from build123d import *

# Parameters (mm, degrees)
SKETCH1_W           = 63.75
SKETCH1_H           = 36.5
BOSS_EXTRUDE1_DEPTH = 1
SKETCH2_W           = 63.75
SKETCH2_H           = 1
BOSS_EXTRUDE2_DEPTH = 15
BOSS_EXTRUDE3_DEPTH = 1
CUT_EXTRUDE1_REACH  = 18


with BuildPart() as part:
    # Sketch1 → Boss-Extrude1 (new body)
    with BuildSketch(Plane(origin=(0, 0, 0), x_dir=(1, 0, 0), z_dir=(0, 1, 0))):
        Rectangle(SKETCH1_W, SKETCH1_H)
    extrude(amount=-BOSS_EXTRUDE1_DEPTH)

    # Sketch2 → Boss-Extrude2 (add)
    with BuildSketch(Plane(origin=(0, -1, 0), x_dir=(-1, 0, 0), z_dir=(0, -1, 0))):
        with Locations((0, -17.75)):
            Rectangle(SKETCH2_W, SKETCH2_H)
    extrude(amount=BOSS_EXTRUDE2_DEPTH)

    # Sketch3 → Boss-Extrude3 (add)
    with BuildSketch(Plane.XY.offset(18.25)):
        Polygon((-31.875, 0), (31.875, 0), (31.875, -1), (29.875, -1), (29.875, -16), (-29.875, -16), (-29.875, -1), (-31.875, -1), align=None)
    extrude(amount=BOSS_EXTRUDE3_DEPTH)

    # Sketch4 → Cut-Extrude1 (cut, up to next)
    with BuildSketch(Plane(origin=(0, 0, 0), x_dir=(1, 0, 0), z_dir=(0, 1, 0)), mode=Mode.PRIVATE) as cut_extrude1_sk1:
        with BuildLine():
            Line((-23.706953695, -13.257748955), (-24.425558305, -12.539144346))
            ThreePointArc((-24.425558305, -12.539144346), (-25.839771867, -12.539144346), (-25.839771867, -13.953357908))
            Line((-25.839771867, -13.953357908), (-25.121167258, -14.671962518))
            ThreePointArc((-25.121167258, -14.671962518), (-23.706953695, -14.671962518), (-23.706953695, -13.257748955))
        make_face()
    cut_extrude1_tool1 = extrude(cut_extrude1_sk1.sketch, amount=-CUT_EXTRUDE1_REACH, mode=Mode.PRIVATE) & part.part
    add(cut_extrude1_tool1.solids().sort_by_distance((-24.773363, 0, 13.605553))[0], mode=Mode.SUBTRACT)
    # Sketch4 → Cut-Extrude1 (cut, up to next)
    with BuildSketch(Plane(origin=(0, 0, 0), x_dir=(1, 0, 0), z_dir=(0, 1, 0)), mode=Mode.PRIVATE) as cut_extrude1_sk2:
        with BuildLine():
            Line((-18.612300872, -13.743096131), (-24.910905481, -7.444491522))
            ThreePointArc((-24.910905481, -7.444491522), (-26.325119043, -7.444491522), (-26.325119043, -8.858705084))
            Line((-26.325119043, -8.858705084), (-20.026514434, -15.157309694))
            ThreePointArc((-20.026514434, -15.157309694), (-18.612300872, -15.157309694), (-18.612300872, -13.743096131))
        make_face()
    cut_extrude1_tool2 = extrude(cut_extrude1_sk2.sketch, amount=-CUT_EXTRUDE1_REACH, mode=Mode.PRIVATE) & part.part
    add(cut_extrude1_tool2.solids().sort_by_distance((-22.46871, 0, 11.300901))[0], mode=Mode.SUBTRACT)
    # Sketch4 → Cut-Extrude1 (cut, up to next)
    with BuildSketch(Plane(origin=(0, 0, 0), x_dir=(1, 0, 0), z_dir=(0, 1, 0)), mode=Mode.PRIVATE) as cut_extrude1_sk3:
        with BuildLine():
            Line((-12.983889235, -13.694684495), (-24.862493845, -1.816079885))
            ThreePointArc((-24.862493845, -1.816079885), (-26.276707407, -1.816079885), (-26.276707407, -3.230293448))
            Line((-26.276707407, -3.230293448), (-14.398102798, -15.108898057))
            ThreePointArc((-14.398102798, -15.108898057), (-12.983889235, -15.108898057), (-12.983889235, -13.694684495))
        make_face()
    cut_extrude1_tool3 = extrude(cut_extrude1_sk3.sketch, amount=-CUT_EXTRUDE1_REACH, mode=Mode.PRIVATE) & part.part
    add(cut_extrude1_tool3.solids().sort_by_distance((-19.630298, 0, 8.462489))[0], mode=Mode.SUBTRACT)
    # Sketch4 → Cut-Extrude1 (cut, up to next)
    with BuildSketch(Plane(origin=(0, 0, 0), x_dir=(1, 0, 0), z_dir=(0, 1, 0)), mode=Mode.PRIVATE) as cut_extrude1_sk4:
        with BuildLine():
            Line((-7.19192546, -13.482720719), (-24.650530069, 3.97588389))
            ThreePointArc((-24.650530069, 3.97588389), (-26.064743631, 3.97588389), (-26.064743631, 2.561670328))
            Line((-26.064743631, 2.561670328), (-8.606139022, -14.896934282))
            ThreePointArc((-8.606139022, -14.896934282), (-7.19192546, -14.896934282), (-7.19192546, -13.482720719))
        make_face()
    cut_extrude1_tool4 = extrude(cut_extrude1_sk4.sketch, amount=-CUT_EXTRUDE1_REACH, mode=Mode.PRIVATE) & part.part
    add(cut_extrude1_tool4.solids().sort_by_distance((-16.628335, 0, 5.460525))[0], mode=Mode.SUBTRACT)
    # Sketch4 → Cut-Extrude1 (cut, up to next)
    with BuildSketch(Plane(origin=(0, 0, 0), x_dir=(1, 0, 0), z_dir=(0, 1, 0)), mode=Mode.PRIVATE) as cut_extrude1_sk5:
        with BuildLine():
            Line((-1.598647721, -13.469442981), (-24.63725233, 9.569161629))
            ThreePointArc((-24.63725233, 9.569161629), (-26.051465893, 9.569161629), (-26.051465893, 8.154948066))
            Line((-26.051465893, 8.154948066), (-3.012861283, -14.883656543))
            ThreePointArc((-3.012861283, -14.883656543), (-1.598647721, -14.883656543), (-1.598647721, -13.469442981))
        make_face()
    cut_extrude1_tool5 = extrude(cut_extrude1_sk5.sketch, amount=-CUT_EXTRUDE1_REACH, mode=Mode.PRIVATE) & part.part
    add(cut_extrude1_tool5.solids().sort_by_distance((-13.825057, 0, 2.657247))[0], mode=Mode.SUBTRACT)
    # Sketch4 → Cut-Extrude1 (cut, up to next)
    with BuildSketch(Plane(origin=(0, 0, 0), x_dir=(1, 0, 0), z_dir=(0, 1, 0)), mode=Mode.PRIVATE) as cut_extrude1_sk6:
        with BuildLine():
            Line((3.848599736, -13.602195524), (-24.770004873, 15.016409086))
            ThreePointArc((-24.770004873, 15.016409086), (-26.184218436, 15.016409086), (-26.184218436, 13.602195524))
            Line((-26.184218436, 13.602195524), (2.434386174, -15.016409086))
            ThreePointArc((2.434386174, -15.016409086), (3.848599736, -15.016409086), (3.848599736, -13.602195524))
        make_face()
    cut_extrude1_tool6 = extrude(cut_extrude1_sk6.sketch, amount=-CUT_EXTRUDE1_REACH, mode=Mode.PRIVATE) & part.part
    add(cut_extrude1_tool6.solids().sort_by_distance((-11.167809, 0, 0))[0], mode=Mode.SUBTRACT)
    # Sketch4 → Cut-Extrude1 (cut, up to next)
    with BuildSketch(Plane(origin=(0, 0, 0), x_dir=(1, 0, 0), z_dir=(0, 1, 0)), mode=Mode.PRIVATE) as cut_extrude1_sk7:
        with BuildLine():
            Line((9.432504411, -13.602195524), (-19.186100198, 15.016409086))
            ThreePointArc((-19.186100198, 15.016409086), (-20.600313761, 15.016409086), (-20.600313761, 13.602195524))
            Line((-20.600313761, 13.602195524), (8.018290849, -15.016409086))
            ThreePointArc((8.018290849, -15.016409086), (9.432504411, -15.016409086), (9.432504411, -13.602195524))
        make_face()
    cut_extrude1_tool7 = extrude(cut_extrude1_sk7.sketch, amount=-CUT_EXTRUDE1_REACH, mode=Mode.PRIVATE) & part.part
    add(cut_extrude1_tool7.solids().sort_by_distance((-5.583905, 0, 0))[0], mode=Mode.SUBTRACT)
    # Sketch4 → Cut-Extrude1 (cut, up to next)
    with BuildSketch(Plane(origin=(0, 0, 0), x_dir=(1, 0, 0), z_dir=(0, 1, 0)), mode=Mode.PRIVATE) as cut_extrude1_sk8:
        with BuildLine():
            Line((15.016409086, -13.602195524), (-13.602195524, 15.016409086))
            ThreePointArc((-13.602195524, 15.016409086), (-15.016409086, 15.016409086), (-15.016409086, 13.602195524))
            Line((-15.016409086, 13.602195524), (13.602195524, -15.016409086))
            ThreePointArc((13.602195524, -15.016409086), (15.016409086, -15.016409086), (15.016409086, -13.602195524))
        make_face()
    cut_extrude1_tool8 = extrude(cut_extrude1_sk8.sketch, amount=-CUT_EXTRUDE1_REACH, mode=Mode.PRIVATE) & part.part
    add(cut_extrude1_tool8.solids().sort_by_distance((0, 0, 0))[0], mode=Mode.SUBTRACT)
    # Sketch4 → Cut-Extrude1 (cut, up to next)
    with BuildSketch(Plane(origin=(0, 0, 0), x_dir=(1, 0, 0), z_dir=(0, 1, 0)), mode=Mode.PRIVATE) as cut_extrude1_sk9:
        with BuildLine():
            Line((20.596409086, -13.602195524), (-8.022195524, 15.016409086))
            ThreePointArc((-8.022195524, 15.016409086), (-9.436409086, 15.016409086), (-9.436409086, 13.602195524))
            Line((-9.436409086, 13.602195524), (19.182195524, -15.016409086))
            ThreePointArc((19.182195524, -15.016409086), (20.596409086, -15.016409086), (20.596409086, -13.602195524))
        make_face()
    cut_extrude1_tool9 = extrude(cut_extrude1_sk9.sketch, amount=-CUT_EXTRUDE1_REACH, mode=Mode.PRIVATE) & part.part
    add(cut_extrude1_tool9.solids().sort_by_distance((5.58, 0, 0))[0], mode=Mode.SUBTRACT)
    # Sketch4 → Cut-Extrude1 (cut, up to next)
    with BuildSketch(Plane(origin=(0, 0, 0), x_dir=(1, 0, 0), z_dir=(0, 1, 0)), mode=Mode.PRIVATE) as cut_extrude1_sk10:
        with BuildLine():
            Line((26.184121966, -13.602099067), (-2.442291993, 15.016505543))
            ThreePointArc((-2.442291993, 15.016505543), (-3.856505543, 15.016312616), (-3.856312616, 13.602099067))
            Line((-3.856312616, 13.602099067), (24.770101343, -15.016505543))
            ThreePointArc((24.770101343, -15.016505543), (26.184314892, -15.016312616), (26.184121966, -13.602099067))
        make_face()
    cut_extrude1_tool10 = extrude(cut_extrude1_sk10.sketch, amount=-CUT_EXTRUDE1_REACH, mode=Mode.PRIVATE) & part.part
    add(cut_extrude1_tool10.solids().sort_by_distance((11.163905, 0, 0))[0], mode=Mode.SUBTRACT)
    # Sketch4 → Cut-Extrude1 (cut, up to next)
    with BuildSketch(Plane(origin=(0, 0, 0), x_dir=(1, 0, 0), z_dir=(0, 1, 0)), mode=Mode.PRIVATE) as cut_extrude1_sk11:
        with BuildLine():
            Line((26.184218436, -8.030004873), (3.137804476, 15.016409086))
            ThreePointArc((3.137804476, 15.016409086), (1.723590914, 15.016409086), (1.723590914, 13.602195524))
            Line((1.723590914, 13.602195524), (24.770004873, -9.444218436))
            ThreePointArc((24.770004873, -9.444218436), (26.184218436, -9.444218436), (26.184218436, -8.030004873))
        make_face()
    cut_extrude1_tool11 = extrude(cut_extrude1_sk11.sketch, amount=-CUT_EXTRUDE1_REACH, mode=Mode.PRIVATE) & part.part
    add(cut_extrude1_tool11.solids().sort_by_distance((13.953905, 0, -2.786095))[0], mode=Mode.SUBTRACT)
    # Sketch4 → Cut-Extrude1 (cut, up to next)
    with BuildSketch(Plane(origin=(0, 0, 0), x_dir=(1, 0, 0), z_dir=(0, 1, 0)), mode=Mode.PRIVATE) as cut_extrude1_sk12:
        with BuildLine():
            Line((26.184218436, -2.450004873), (8.717804476, 15.016409086))
            ThreePointArc((8.717804476, 15.016409086), (7.303590914, 15.016409086), (7.303590914, 13.602195524))
            Line((7.303590914, 13.602195524), (24.770004873, -3.864218436))
            ThreePointArc((24.770004873, -3.864218436), (26.184218436, -3.864218436), (26.184218436, -2.450004873))
        make_face()
    cut_extrude1_tool12 = extrude(cut_extrude1_sk12.sketch, amount=-CUT_EXTRUDE1_REACH, mode=Mode.PRIVATE) & part.part
    add(cut_extrude1_tool12.solids().sort_by_distance((16.743905, 0, -5.576095))[0], mode=Mode.SUBTRACT)
    # Sketch4 → Cut-Extrude1 (cut, up to next)
    with BuildSketch(Plane(origin=(0, 0, 0), x_dir=(1, 0, 0), z_dir=(0, 1, 0)), mode=Mode.PRIVATE) as cut_extrude1_sk13:
        with BuildLine():
            Line((26.184218436, 3.129995127), (14.297804476, 15.016409086))
            ThreePointArc((14.297804476, 15.016409086), (12.883590914, 15.016409086), (12.883590914, 13.602195524))
            Line((12.883590914, 13.602195524), (24.770004873, 1.715781564))
            ThreePointArc((24.770004873, 1.715781564), (26.184218436, 1.715781564), (26.184218436, 3.129995127))
        make_face()
    cut_extrude1_tool13 = extrude(cut_extrude1_sk13.sketch, amount=-CUT_EXTRUDE1_REACH, mode=Mode.PRIVATE) & part.part
    add(cut_extrude1_tool13.solids().sort_by_distance((19.533905, 0, -8.366095))[0], mode=Mode.SUBTRACT)
    # Sketch4 → Cut-Extrude1 (cut, up to next)
    with BuildSketch(Plane(origin=(0, 0, 0), x_dir=(1, 0, 0), z_dir=(0, 1, 0)), mode=Mode.PRIVATE) as cut_extrude1_sk14:
        with BuildLine():
            Line((26.369863641, 8.895640332), (20.063449682, 15.202054291))
            ThreePointArc((20.063449682, 15.202054291), (18.64923612, 15.202054291), (18.64923612, 13.787840729))
            Line((18.64923612, 13.787840729), (24.955650079, 7.48142677))
            ThreePointArc((24.955650079, 7.48142677), (26.369863641, 7.48142677), (26.369863641, 8.895640332))
        make_face()
    cut_extrude1_tool14 = extrude(cut_extrude1_sk14.sketch, amount=-CUT_EXTRUDE1_REACH, mode=Mode.PRIVATE) & part.part
    add(cut_extrude1_tool14.solids().sort_by_distance((22.50955, 0, -11.341741))[0], mode=Mode.SUBTRACT)
    # Sketch4 → Cut-Extrude1 (cut, up to next)
    with BuildSketch(Plane(origin=(0, 0, 0), x_dir=(1, 0, 0), z_dir=(0, 1, 0)), mode=Mode.PRIVATE) as cut_extrude1_sk15:
        with BuildLine():
            Line((26.184218436, 14.289995127), (25.457804476, 15.016409086))
            ThreePointArc((25.457804476, 15.016409086), (24.043590914, 15.016409086), (24.043590914, 13.602195524))
            Line((24.043590914, 13.602195524), (24.770004873, 12.875781564))
            ThreePointArc((24.770004873, 12.875781564), (26.184218436, 12.875781564), (26.184218436, 14.289995127))
        make_face()
    cut_extrude1_tool15 = extrude(cut_extrude1_sk15.sketch, amount=-CUT_EXTRUDE1_REACH, mode=Mode.PRIVATE) & part.part
    add(cut_extrude1_tool15.solids().sort_by_distance((25.113905, 0, -13.946095))[0], mode=Mode.SUBTRACT)


solid = part.part
Could you check a few things on this model? Use its own coordinates, in mm. A direction names the side the tool comes from. Round coordinates to 2 decimals unless told otherwise and drop trailing zeros. Order: outer loops, then holes, each group sorted by start corner. A loop starts at its lowest first (then second) coordinate and runs counter-clockwise, first axis right, second up. Notation, with made-up numbers: M -32,65 L -22,65 A13 ccw -22,90 Z; hole C 13.5,46.25 d3. An arc over 180 degrees is marked long. One line per item, written item: value.
(1) If we mould it in two halves opening along X, with no side actions, what happens to faces 1 (the flat face through (-15.799, -0.493, 4.876)), 2 (the flat face through (31, -8, 18.25))? For each: released by +X, released by -X, zero draft, split by the parting line, or undercut.
Ans:
face 1: undercut
face 2: zero draft
(2) Imagine slicing it at B-B (x = -5). Write out the boundary of the cut face in (y, z).
Ans:
outline: M -16,17.25 L -1,17.25 L -1,12.9 L 0,12.9 L 0,19.25 L -16,19.25 Z; M -1,-18.25 L 0,-18.25 L 0,-11.99 L -1,-11.99 Z; M -1,-9.17 L 0,-9.17 L 0,-6.41 L -1,-6.41 Z; M -1,-3.59 L 0,-3.59 L 0,-0.83 L -1,-0.83 Z; M -1,2 L 0,2 L 0,4.75 L -1,4.75 Z; M -1,7.58 L 0,7.58 L 0,10.07 L -1,10.07 Z
(3) Which directions (+Z, -Z, +X, -X, +Y, -Y) give clear straight access to the entire face, cutting with the end or side of a thin tool? Please do faces 3 (the flat face through (20.324, -0.493, -8.99)), 4 (the flat face through (0, -16, 18)), 5 (the flat face through (0, -8, 17.25)).
Ans:
face 3: +Y, -Y
face 4: +Z, -Z, +X, -X, -Y
face 5: -Z, +X, -X, -Y
(4) I need wall thicknesses on line 1 along Y through (x, z) = (3.5, -10); line 2 along Z through (x, y) = (17.5, -13.75). Which ranges of each line are inside material? Lowest first, please. Write a range as from..to.
Ans:
line 1: y = -1..0
line 2: z = 17.25..19.25
(5) Imagine slicing it at A-A (y = -4.25). Write out the boundary of the cut face in (x, z) (3 decimals), and give its area (4 significant figures).
Ans:
outline: M -31.875,17.25 L 31.875,17.25 L 31.875,18.25 L 29.875,18.25 L 29.875,19.25 L -29.875,19.25 L -29.875,18.25 L -31.875,18.25 Z
area: 123.5 mm^2
(6) I'm going to push flat-ended pins straight in: P1, Ø0.5, axis at x = -30.5, z = 19, coming from the -Y side; P2, Ø0.8, axis at y = -11.5, z = 19, coming from the +X side (3 decimals); P3, Ø6, axis at y = -5.5, z = 5.5, coming from the -X side; P4, Ø1, axis at x = 31.5, y = -10, coming from the +Z side. Where does each tip first touch, or does it pass through?
Ans:
P1: stops at y = -1
P2: stops at x = 29.875
P3: passes through
P4: stops at z = 18.25
(7) Imagine slicing it at C-C (z = -11.5). Count the separate pieces of the cut face and the enclosed holes in it, and give its area (3 significant figures).
Ans:
separate pieces: 10
enclosed holes: 0
area: 38.3 mm^2
